Geometry check sheet. Reference: the model listing, model coordinates, mm. A direction names the side the tool comes from. Coordinates: 2 decimals unless noted, no trailing zeros. Write each loop counter-clockwise with the first axis right and the second up, starting at its lowest first coordinate (ties: lowest second). Pieces come first, ordered by that corner, then holes. Notation, with made-up numbers: (-20.5, -9.5) -> (-12.5, -9.5) arc R31 cw to (-12.5, 27.5) -> close; hole circle Ø7 at (33, 51.25). An arc over 180 degrees is marked (long way). Answer in a Markdown table with one row per item. Add a question column.
1. Cross-section at A-A on x = -14. Record the cut outline in (y, z) (3 decimals).
2. Scan lines: L1, parallel to Y at x = -14, z = -1.05 (3 decimals); L2, parallel to Y at x = 17, z = -0.8 (3 decimals); L3, parallel to Z at x = -15, y = -12.5. Record each from-to range of solid material in increasing order. Write a range as from..to.
3. Depth check by flat-ended pin: P1, Ø1.9, axis at x = 3.5, z = -5.5, coming from the +Y side; P2, Ø3.5, axis at x = -14, y = 14, coming from the +Z side; P3, Ø19, axis at x = 2.5, y = 4.5, coming from the -Z side. Enter the tip coordinate at first touch or a pass-through.
4. Set-up check for faces 1 (the cylindrical face through (12.25, -0.05, 3.01)), 2 (the flat face through (-8, -5, 3)), 3 (the flat face through (9, -2.25, 3)), 4 (the flat face through (5, -11, -5)): record each of +Z, -Z, +X, -X, +Y, -Y from which the full face is reachable in a straight line by a thin tool's end or side.
5. Mould release check, pull along X, two halves, no side actions. Record for faces 5 (the cylindrical face through (14.519, -14.998, -0.789)), 6 (the flat face through (0, -8, 3)), 7 (the cylindrical face through (17.6, -16.05, -0.79)), 8 (the flat face through (-19.05, 0, -1)): pulls with the +X half, pulls with the -X half, needs draft (parallel to the pull), parting line crosses it, or undercut.
6. Cross-section at D-D on x = 9.5. Record the cut outline in (y, z), and give its area (3 significant figures).
7. Cross-section at C-C on y = 0. Record the cut outline in (x, z), and give its area (3 significant figures).
```python
from build123d import *

# Parameters (mm, degrees)
SKETCH_W     = 38.1
SKETCH_H     = 38.1
SKETCH_R     = 1.125
PAD_DEPTH    = 1.6
PAD001_DEPTH = 6.1
SKETCH002_R  = 7.5
PAD002_DEPTH = 1
SKETCH003_W  = 10
SKETCH003_H  = 4.5
PAD003_DEPTH = 6.25


with BuildPart() as part:
    # Sketch → Pad (new body)
    with BuildSketch(Plane.XY):
        Rectangle(SKETCH_W, SKETCH_H)
        with Locations((-14, 14)):
            Circle(SKETCH_R, mode=Mode.SUBTRACT)
        with Locations((14, 14)):
            Circle(SKETCH_R, mode=Mode.SUBTRACT)
        with Locations((14, -14)):
            Circle(SKETCH_R, mode=Mode.SUBTRACT)
        with Locations((-14, -14)):
            Circle(SKETCH_R, mode=Mode.SUBTRACT)
        with Locations((-17, 17)):
            Circle(SKETCH_R, mode=Mode.SUBTRACT)
        with Locations((17, 17)):
            Circle(SKETCH_R, mode=Mode.SUBTRACT)
        with Locations((17, -17)):
            Circle(SKETCH_R, mode=Mode.SUBTRACT)
        with Locations((-17, -17)):
            Circle(SKETCH_R, mode=Mode.SUBTRACT)
    extrude(amount=-PAD_DEPTH)

    # Sketch001 → Pad001 (join)
    with BuildSketch(Plane.XY):
        with BuildLine():
            Line((-8, 2.25), (-8, 8))
            Line((-8, 8), (8, 8))
            Line((8, 8), (8, 2.25))
            Line((8, 2.25), (10.000011, 2.25))
            ThreePointArc((10.000011, -2.25), (12.25, 0), (10.000011, 2.25))
            Line((8, -2.25), (10.000011, -2.25))
            Line((8, -8), (8, -2.25))
            Line((-8, -8), (8, -8))
            Line((-8, -2.25), (-8, -8))
            Line((-9.999989, -2.25), (-8, -2.25))
            ThreePointArc((-10, 2.25), (-12.25, -6e-06), (-9.999989, -2.25))
            Line((-10, 2.25), (-8, 2.25))
        make_face()
    extrude(amount=PAD001_DEPTH)

    # Sketch002 (on DatumPlane) → Pad002 (join)
    with BuildSketch(Plane.XY.offset(6.1)):
        Circle(SKETCH002_R)
    extrude(amount=PAD002_DEPTH)

    # Sketch003 (on DatumPlane) → Pad003 (join)
    with BuildSketch(Plane(origin=(0, 0, -1.6), x_dir=(1, 0, 0), z_dir=(0, 0, -1))):
        with Locations((5, 13.25)):
            Rectangle(SKETCH003_W, SKETCH003_H)
    extrude(amount=PAD003_DEPTH)


solid = part.part
```
Results found:
| question | item | result |
|---|---|---|
| 1 | outline | (-19.05, -1.6) -> (-15.125, -1.6) -> (-15.125, 0) -> (-19.05, 0) -> close; (-12.875, -1.6) -> (12.875, -1.6) -> (12.875, 0) -> (-12.875, 0) -> close; (15.125, -1.6) -> (19.05, -1.6) -> (19.05, 0) -> (15.125, 0) -> close |
| 2 | L1 | y = -19.05..-15.125, -12.875..12.875, 15.125..19.05 |
| 2 | L2 | y = -19.05..-18.125, -15.875..15.875, 18.125..19.05 |
| 2 | L3 | z = -1.6..0 |
| 3 | P1 | stops at y = -11 |
| 3 | P2 | stops at z = 0 |
| 3 | P3 | stops at z = -1.6 |
| 4 | face 1 | +Z, +X |
| 4 | face 2 | +Z, -X, -Y |
| 4 | face 3 | +Z, +X, -Y |
| 4 | face 4 | -Z, +X, -X, +Y |
| 5 | face 5 | undercut |
| 5 | face 6 | needs draft |
| 5 | face 7 | undercut |
| 5 | face 8 | pulls with the -X half |
| 6 | outline | (-19.05, -1.6) -> (-15.5, -1.6) -> (-15.5, -7.85) -> (-11, -7.85) -> (-11, -1.6) -> (19.05, -1.6) -> (19.05, 0) -> (2.25, 0) -> (2.25, 6.1) -> (-2.25, 6.1) -> (-2.25, 0) -> (-19.05, 0) -> close |
| 6 | area | 117 mm^2 |
| 7 | outline | (-19.05, -1.6) -> (19.05, -1.6) -> (19.05, 0) -> (12.25, 0) -> (12.25, 6.1) -> (7.5, 6.1) -> (7.5, 7.1) -> (-7.5, 7.1) -> (-7.5, 6.1) -> (-12.25, 6.1) -> (-12.25, 0) -> (-19.05, 0) -> close |
| 7 | area | 225 mm^2 |
